Can you work these out from the model? Positions are in its coordinate system, mm. A direction names the side the tool comes from. Give positions to 0.01 mm unless a question says otherwise; leave off trailing zeros. Loops run counter-clockwise (first coordinate to the right, second up) from the corner with the lowest first, then second, coordinate; pieces in that order, holes last. Notation, with made-up numbers: (8.5, -39) -> (52.5, -39) arc R20 ccw to (52.5, -16) -> close; hole circle Ø9 at (41, 72). An arc over 180 degrees is marked (long way). One line per question, with ' | ' between items.
Autodesk Inventor part; units mm, degrees
ref_plane "YZ Plane" through (0, 0, 0) normal (1, 0, 0) x (0, 1, 0)
ref_plane "XZ Plane" through (0, 0, 0) normal (0, 1, 0) x (-1, 0, 0)
ref_plane "XY Plane" through (0, 0, 0) normal (0, 0, 1) x (1, 0, 0)
sketch "Эскиз1" plane through (0, 0, 0) normal (0, 0, 1) x (1, 0, 0)
  circle A0 centre (0, 0) radius 37.5
  circle A1 centre (0, 0) radius 2.1
  circle A2 centre (-8, 0) radius 2.1
  circle A3 centre (8, 0) radius 2.1
  line L0 (0, 0) -> (21.2822, 0) construction
  line L1 (0, 0) -> (-18.9176, 0) construction
  dimension "d0" = 75
  dimension "d1" = 4.2
  dimension "d2" = 4.2
  dimension "d3" = 4.2
  dimension "d4" = 8
  dimension "d5" = 8
extrude "Выдавливание1" add sketch "Эскиз1" along normal blind 4
sketch "Эскиз2" plane through (0, 0, 4) normal (0, 0, 1) x (1, 0, 0)
  circle A0 centre (0, 0) radius 2.1
  line L0 (0, 0) -> (0, -140) construction
  line L1 (-20, -20) -> (-20, -65.8579)
  arc A1 (20, -20) -> (-20, -20) centre (0, -20) ccw
  line L2 (0, -70) -> (64.1421, -134.1421) construction
  line L3 (0, -98.2843) -> (35.8579, -134.1421)
  line L4 (64.1421, -105.8579) -> (28.2843, -70)
  arc A2 (35.8579, -134.1421) -> (64.1421, -105.8579) centre (50, -120) ccw
  line L5 (0, -70) -> (90.7107, -70) construction
  line L6 (0, -140) -> (114.1632, -140) construction
  line L7 (0, -98.2843) -> (-11.2132, -87.0711)
  arc A3 (-20, -65.8579) -> (-11.2132, -87.0711) centre (10, -65.8579) ccw
  line L8 (28.2843, -70) -> (28.7868, -70.5025)
  line L9 (20, -49.2893) -> (20, -20)
  arc A4 (20, -49.2893) -> (28.7868, -70.5025) centre (50, -49.2893) ccw
  point P0 (32.0711, -102.0711)
  point P1 (2.0971, -0.1103)
  point P2 (-2.0971, -0.1102)
  dimension "d19" = 45
  dimension "d20" = 40
  dimension "d21" = 30
  dimension "d22" = 30
extrude "Выдавливание2" add sketch "Эскиз2" against normal blind 4 contours A0 A1 L9 A4 L4 A2 L3 L7 A3 L1
fillet "Сопряжение1" radius 10 2 edges at (-20, -31.7214, 2) (20, -31.7214, 2)
Q1. For pin 1 Ø3.5 at (x, y) = (0, 0) entering from -Z, with a flat end and sliding along its axis, tell me the tip position at first contact or that it passes through.
Entries:
pin 1: through
Q2. On a 3-axis mill with a long thin cutter (end or side, diameter ignored), from which of +Z, -Z, +X, -X, +Y, -Y can I reach the whole of each face in a straight line? I mean faces 1 (the face through (20, -43, 2)), 2 (the face through (-1.29, 37.478, 1.972)), 3 (the face through (-20, -51, 2)). Say none if no direction works.
Entries:
face 1: +Z, -Z, +X | face 2: +Z, -Z | face 3: +Z, -Z, -X, -Y
Q3. If we mould it in two halves opening along X, with no side actions, what happens to faces 4 (the face through (-20.995, -32.479, 1.972)), 5 (the face through (20.94, -32.59, 1.97)), 6 (the face through (8.713, 1.975, 1.972))? For each: pulls with the +X half, pulls with the -X half, needs draft (parallel to the pull), parting line crosses it, or undercut.
Entries:
face 4: pulls with the -X half | face 5: pulls with the +X half | face 6: undercut
Q4. If we section it at B-B (y = -41): Write out the boundary of the cut face in (x, z).
Entries:
outline: (-20, 0) -> (20, 0) -> (20, 4) -> (-20, 4) -> close
Q5. If I drill on probe 1 along X at (y, z) = (0, 1.1); probe 2 along Y at (x, z) = (0, 0.95); probe 3 along Y at (x, z) = (24, 3.5), over which ranges is the centre line in solid material (lowest first)? Write a range as from..to.
Entries:
probe 1: -37.5..-10.1, -5.9..-2.1, 2.1..5.9, 10.1..37.5 | probe 2: -98.28..-2.1, 2.1..37.5 | probe 3: -122.28..-64.26, -28.81..28.81
Q6. If we section it at C-C (x = 4): Write out the boundary of the cut face in (y, z).
Entries:
outline: (-102.28, 0) -> (37.29, 0) -> (37.29, 4) -> (-102.28, 4) -> close
Q7. If we section it at A-A (z = 3.35): Write out the boundary of the cut face in (x, y).
Entries:
outline: (-23.68, -29.07) arc R10 cw to (-20, -36.83) -> (-20, -65.86) arc R30 ccw to (-11.21, -87.07) -> (0, -98.28) -> (35.86, -134.14) arc R20 ccw to (64.14, -105.86) -> (28.79, -70.5) arc R30 cw to (20, -49.29) -> (20, -36.83) arc R10 cw to (23.68, -29.07) arc R37.5 ccw (long way) to start; hole (-8.69, -1.98) arc R20 cw to (-6.13, -0.96) arc R2.1 ccw (long way) to start; hole circle Ø4.2 at (0, 0); hole (6.13, -0.96) arc R20 cw to (8.69, -1.98) arc R2.1 ccw (long way) to start
